Answer from the drawing. Dimensions are ordinates in mm from the lowest x, y and z of the part. Give positions to 0.01 mm unless a question says otherwise; leave off trailing zeros. Loops run counter-clockwise (first coordinate to the right, second up) from the corner with the lowest first, then second, coordinate; pieces in that order, holes last.
(1) Find section C-C, the plane x = 26. Write down the section's boundary in (y, z), then the cut area to 3 significant figures.
(2) Straight lines are drawn through the part: probe 1 along X at (y, z) = (2.25, 1.25); probe 2 along X at (y, z) = (1, 3.5); probe 3 along Y at (x, z) = (25.5, 4.25). For each, find the intervals that lie inside material, in ascending order.
(3) Find section A-A, the plane z = 4. Write down the section's boundary in (x, y), then the cut area to 3 significant figures.
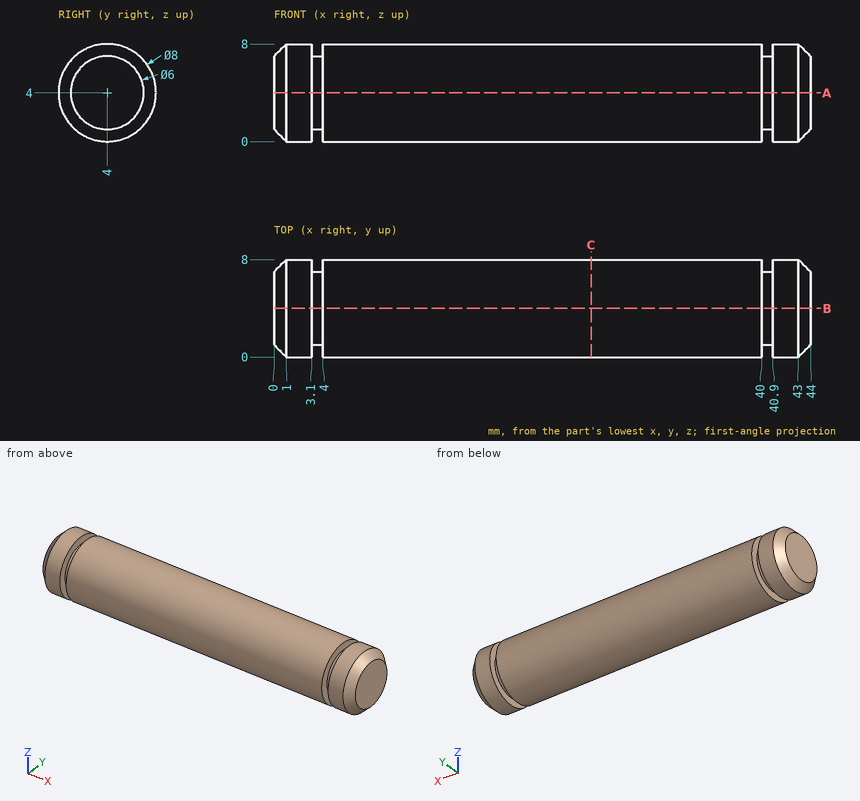
Entries:
1. outline: circle Ø8 at (4, 4)
1. area: 50.3 mm2
2. probe 1: x = 0.26 to 3.1, 4 to 40, 40.9 to 43.74
2. probe 2: x = 0.04 to 3.1, 4 to 40, 40.9 to 43.96
2. probe 3: y = 0.01 to 7.99
3. outline: (0, 1) - (1, 0) - (3.1, 0) - (3.1, 1) - (4, 1) - (4, 0) - (40, 0) - (40, 1) - (40.9, 1) - (40.9, 0) - (43, 0) - (44, 1) - (44, 7) - (43, 8) - (40.9, 8) - (40.9, 7) - (40, 7) - (40, 8) - (4, 8) - (4, 7) - (3.1, 7) - (3.1, 8) - (1, 8) - (0, 7) - close
3. area: 346 mm2
